```python
from build123d import *

# Parameters (mm, degrees)
F0_R     = 4.699
F1_DEPTH = 152.4
F2_R     = 12.7
F3_DEPTH = 6.35
F4_R     = 2.38125
F5_DEPTH = 12.701


with BuildPart() as f1:
    # F0 (on Right) → F1 (new body)
    with BuildSketch(Plane.YZ):
        Circle(F0_R)
    extrude(amount=F1_DEPTH)

    # F2 (on Right) → F3 (join)
    with BuildSketch(Plane.YZ):
        Circle(F2_R)
    extrude(amount=F3_DEPTH)

    # F4 (on Front) → F5 (cut, through all)
    with BuildSketch(Plane.XZ):
        with Locations((114.3, 0)):
            Circle(F4_R)
    extrude(amount=-F5_DEPTH, mode=Mode.SUBTRACT)


solid = f1.part
```
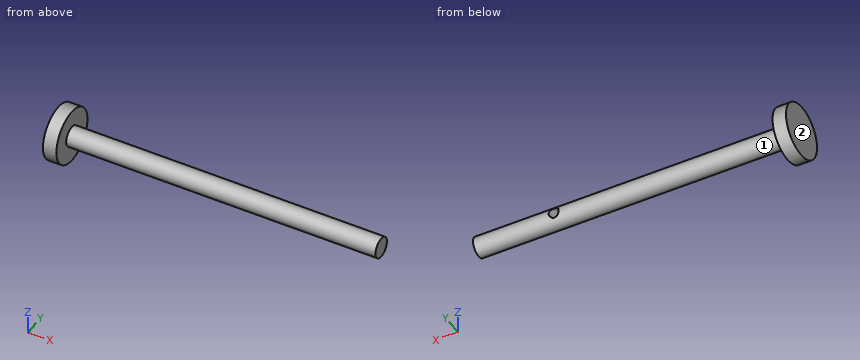
For this review, take the finished solid that the model builds, in its own axes (mm). Face numbers are marked on the shaded views. A direction names the side the tool comes from. Round coordinates to 2 decimals unless told otherwise and drop trailing zeros. Write each loop counter-clockwise with the first axis right and the second up, starting at its lowest first coordinate (ties: lowest second). Pieces come first, ordered by that corner, then holes. Notation, with made-up numbers: M -16.75,85 L 39.25,85 A32 ccw 39.25,113 Z; hole C 68.25,7.25 d4. An arc over 180 degrees is marked long. One line per item, written item: value. Start each with the question number.
(1) We need section A-A (y = 2.5). Give the boundary of the cut face in (x, z).
(2) Insertion check: pin 1 (3 mm diameter, centred on y = 10, z = -4, fed in from -X); pin 2 (7.5 mm diameter, centred on x = 114.3, z = 0, fed in from -Y); pin 3 (5 mm diameter, centred on x = 33.5, y = 1, fed in from +Z); pin 4 (1.5 mm diameter, centred on x = 56.5, y = 3, fed in from +Z). Each pin has a flat end and moves straight along its axis. Give the tip position at first contact, or say it passes through.
(3) We need section D-D (y = -3.25). Give the boundary of the cut face in (x, z).
(4) We need section B-B (z = 0). Give the boundary of the cut face in (x, y).
(5) Wall thickness on line 1 (X direction, y = 3.1, z = 0); line 2 (Z direction, x = 114.3, y = 1.3); line 3 (Z direction, x = 114.3, y = 1.65): over which ranges is each line inside the solid? List them lowest first.
(6) We need section C-C (x = 86). Give the boundary of the cut face in (y, z).
(7) Machinability: for the marked faces 1 and 2, which of the approach directions +Z, -Z, +X, -X, +Y, -Y give a long, thin tool a straight path to every point of the face, cutting with its end or side? Answer none if there is none.
Result:
1. outline: M 0,-12.45 L 6.35,-12.45 L 6.35,-3.98 L 152.4,-3.98 L 152.4,3.98 L 6.35,3.98 L 6.35,12.45 L 0,12.45 Z; hole C 114.3,0 d4.76
2. pin 1: x = 0
2. pin 2: y = -4.7
2. pin 3: z = 4.7
2. pin 4: z = 4.13
3. outline: M 0,-12.28 L 6.35,-12.28 L 6.35,-3.39 L 152.4,-3.39 L 152.4,3.39 L 6.35,3.39 L 6.35,12.28 L 0,12.28 Z
4. outline: M 0,-12.7 L 6.35,-12.7 L 6.35,-4.7 L 152.4,-4.7 L 152.4,4.7 L 116.68,4.7 L 116.68,0 L 111.92,0 L 111.92,4.7 L 6.35,4.7 L 6.35,12.7 L 0,12.7 Z
5. line 1: 0 to 111.92, 116.68 to 152.4
5. line 2: -4.52 to -2.38, 2.38 to 4.52
5. line 3: -4.4 to -2.38, 2.38 to 4.4
6. outline: C 0,0 d9.4
7. face 1: +X
7. face 2: +Z, -Z, -X, +Y, -Y
